Job drawing, mm, ordinate dimensions from the low corner. One solid piece. A direction names the side the tool comes from. Round coordinates to 2 decimals unless told otherwise and drop trailing zeros. Write each loop counter-clockwise with the first axis right and the second up, starting at its lowest first coordinate (ties: lowest second). Pieces come first, ordered by that corner, then holes. Notation, with made-up numbers: (-5.75, -22.75) - (37.25, -22.75) arc R23 ccw to (37.25, -12.75) - close; hole circle Ø2 at (55.5, -3). An arc over 180 degrees is marked (long way). Write each question's results on one line, items separated by ' | '.
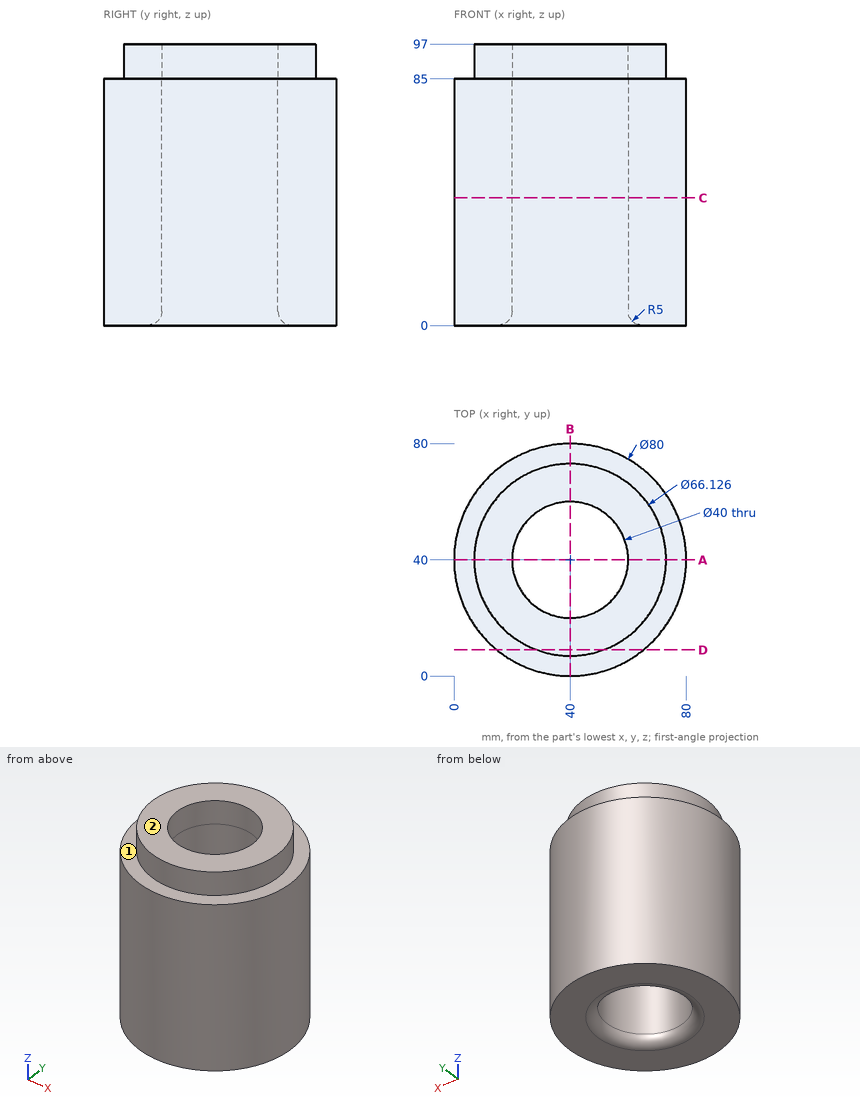
(1) Drill centre lines: probe 1 along Y at (x, z) = (40, 90.25); probe 2 along X at (y, z) = (39, 33) (1 decimal); probe 3 along Z at (x, y) = (14.5, 66.5). Where is each one in solid material? Low to high. Write a range as [from, to].
Worked answers:
probe 1: y = [6.94, 20], [60, 73.06] | probe 2: x = [0, 20], [60, 80] | probe 3: z = [0, 85]
(2) Slice it at A-A, the plane y = 40. Write the cut outline in (x, z).
Worked answers:
outline: (0, 0) - (15, 0) arc R5 ccw to (20, 5) - (20, 97) - (6.94, 97) - (6.94, 85) - (0, 85) - close; (60, 5) arc R5 ccw to (65, 0) - (80, 0) - (80, 85) - (73.06, 85) - (73.06, 97) - (60, 97) - close
(3) Flat gauge pins, fed straight in: pin 1 Ø1.5 at (x, z) = (40, 41) entering from -Y; pin 2 Ø8 at (y, z) = (64.5, 83) entering from +X; pin 3 Ø6 at (x, z) = (65, 45) entering from -Y. Where does each tip first touch, or does it go through?
Worked answers:
pin 1: stops at y = 0 | pin 2: stops at x = 74.35 | pin 3: stops at y = 6.59
(4) Tool access for the marked faces 1 and 2: list every direction of +Z, -Z, +X, -X, +Y, -Y with a clear straight run to the whole face (end or side of a thin tool).
Worked answers:
face 1: +Z | face 2: +Z, +X, -X, +Y, -Y
(5) Slice it at D-D, the plane y = 9. Write the cut outline in (x, z).
Worked answers:
outline: (14.72, 0) - (65.28, 0) - (65.28, 85) - (51.5, 85) - (51.5, 97) - (28.5, 97) - (28.5, 85) - (14.72, 85) - close
(6) Slice it at C-C, the plane z = 44. Write the cut outline in (x, y), and give its area (3 significant figures).
Worked answers:
outline: circle Ø80 at (40, 40); hole circle Ø40 at (40, 40) | area: 3,770 mm2
